Input: dimensioned drawing with shaded views. Units: mm. Origin: part minimum x, y, z. A direction names the side the tool comes from. Give positions to 0.01 mm unless a question says otherwise; leave off trailing zeros. Write each loop counter-clockwise with the first axis right and the second up, starting at its lowest first coordinate (ties: lowest second). Pieces come first, ordered by that corner, then holes. Notation, with made-up numbers: (-33, 31) -> (-27, 31) arc R25 ccw to (-27, 55) -> close; hole circle Ø8 at (-17.5, 19.25). An arc over 180 degrees is marked (long way). Answer in a Markdown table with one row per item. Add a question column.
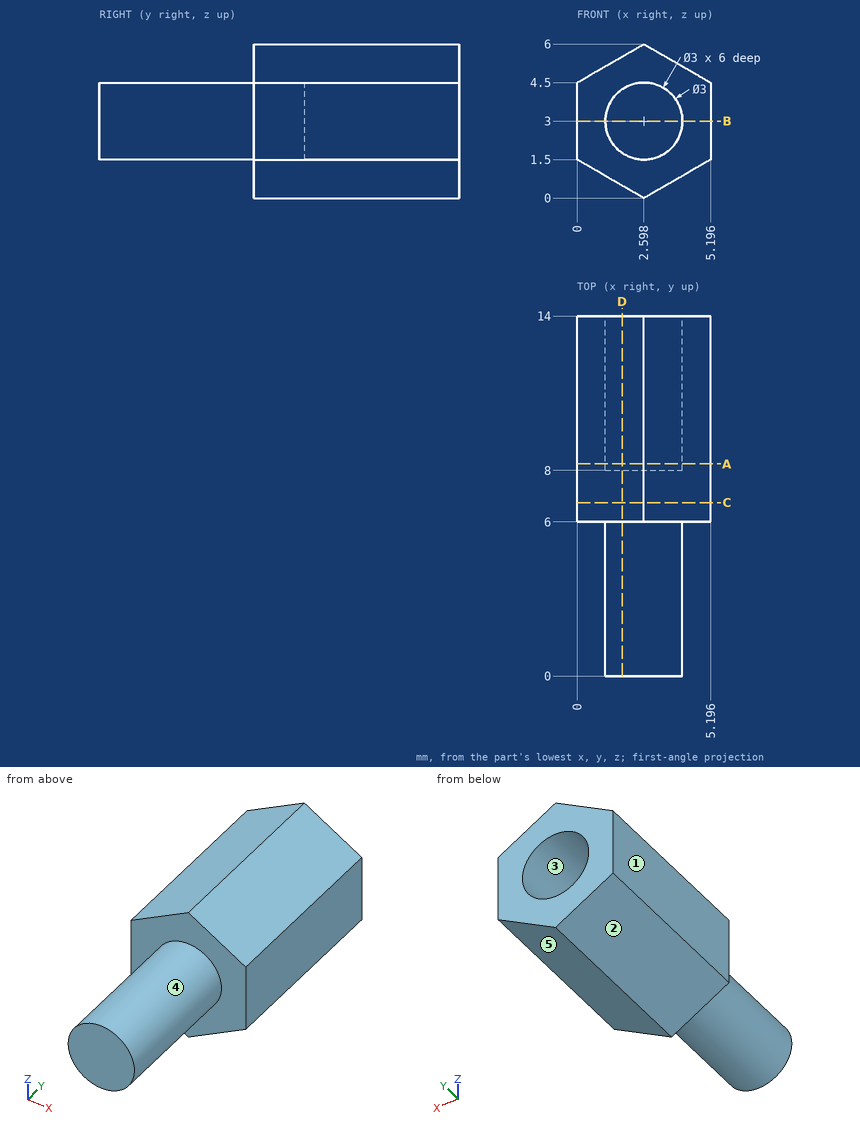
Q1. Section D-D on x = 1.75. Return loops of the section in (y, z).
Q2. Section C-C on y = 6.75. Return loops of the section in (x, z), and give its area (3 significant figures).
Q3. Section A-A on y = 8.25. Return loops of the section in (x, z).
Q4. Access query for the marked faces 4 and 5. Directions: +Z, -Z, +X, -X, +Y, -Y. A direction counts if a zero-diameter tool reaches every point of the face in a straight line with its end or side. Return the directions, or none.
Q5. Section B-B on z = 3. Return loops of the section in (x, y), and give its area (3 significant figures).
Q6. Pull-direction query (Z, two-part tool) for the marked faces 1, 2 and 3; classes: +Z half, -Z half, draft (parallel to the pull), parting line (faces both ways), or undercut.
Q7. Contact query for flat-ended pins moving along their axis: pin 1 Ø1 at (x, y) = (4, 9) entering from -Z; pin 2 Ø1.8 at (x, z) = (2.6, 3) entering from +Y. Output: stop coordinate, or through.
Q8. Line query: probe 1 along X at (y, z) = (9.35, 3); probe 2 along Y at (x, z) = (3.45, 0.6); probe 3 along Y at (x, z) = (2.3, 1.8). Output: solid intervals per line, ascending. Write a range as from..to.
Checks:
| question | item | result |
|---|---|---|
| 1 | outline | (0, 1.76) -> (6, 1.76) -> (6, 0.49) -> (14, 0.49) -> (14, 1.76) -> (8, 1.76) -> (8, 4.24) -> (14, 4.24) -> (14, 5.51) -> (6, 5.51) -> (6, 4.24) -> (0, 4.24) -> close |
| 2 | outline | (0, 1.5) -> (2.6, 0) -> (5.2, 1.5) -> (5.2, 4.5) -> (2.6, 6) -> (0, 4.5) -> close |
| 2 | area | 23.4 mm^2 |
| 3 | outline | (0, 1.5) -> (2.6, 0) -> (5.2, 1.5) -> (5.2, 4.5) -> (2.6, 6) -> (0, 4.5) -> close; hole circle Ø3 at (2.6, 3) |
| 4 | face 4 | -Y |
| 4 | face 5 | -Z, +X, +Y, -Y |
| 5 | outline | (0, 6) -> (1.1, 6) -> (1.1, 0) -> (4.1, 0) -> (4.1, 6) -> (5.2, 6) -> (5.2, 14) -> (4.1, 14) -> (4.1, 8) -> (1.1, 8) -> (1.1, 14) -> (0, 14) -> close |
| 5 | area | 41.6 mm^2 |
| 6 | face 1 | draft |
| 6 | face 2 | -Z half |
| 6 | face 3 | undercut |
| 7 | pin 1 | z = 0.52 |
| 7 | pin 2 | y = 8 |
| 8 | probe 1 | 0..1.1, 4.1..5.2 |
| 8 | probe 2 | 6..14 |
| 8 | probe 3 | 0..8 |
